CAD build for the part. Positions are in the model's coordinates, mm. A direction names the side the tool comes from. Round coordinates to 2 decimals unless told otherwise and drop trailing zeros. Loops run counter-clockwise (first coordinate to the right, second up) from the corner with the lowest first, then second, coordinate; pieces in that order, holes last.
Autodesk Fusion 360 part; units mm, degrees
sketch "Sketch1" plane through (0, 0, 0) normal (0, 0, 1) x (1, 0, 0)
  circle A0 centre (0, 0) radius 16
  circle A1 centre (0, 0) radius 12 construction
  line L0 (0, 0) -> (0, 16) construction
  circle A2 centre (0, 12) radius 2
  circle A3 centre (-12, 0) radius 2
  circle A4 centre (0, -12) radius 2
  circle A5 centre (12, 0) radius 2
  circle A6 centre (0, 0) radius 4
  dimension "d1" = 32
  dimension "d2" = 24
  dimension "d3" = 4
  dimension "d5" = 360
  dimension "d6" = 8
extrude "Extrude1" add sketch "Sketch1" along normal blind 3
sketch "Sketch2" plane through (0, 0, 3) normal (0, 0, 1) x (-1, 0, 0)
  circle A0 centre (0, -12) radius 2
  circle A1 centre (12, 0) radius 2
  circle A2 centre (0, 12) radius 2
  circle A3 centre (-12, 0) radius 2
  circle A4 centre (0, 0) radius 4
  circle A5 centre (0, 0) radius 16
  circle A6 centre (0, 0) radius 8
  dimension "d9" = 16
extrude "Extrude2" add sketch "Sketch2" along normal blind 10 contours A6
ref_plane "WorkPlane1" through (5.6569, -5.6569, 11.1327) normal (0.7071, -0.7071, 0) x (-0.7071, -0.7071, 0)
sketch "Sketch3" plane through (5.6569, -5.6569, 0) normal (0.7071, -0.7071, 0) x (-0.7071, -0.7071, 0)
  line L0 (-8, -13) -> (8, -13)
  line L1 (8, -3) -> (-8, -3)
  line L2 (0, -13) -> (0, -3) construction
  circle A0 centre (0, -8) radius 2
  line L3 (0, -8) -> (0, -10)
  dimension "d13" = 4
  dimension "d14" = 3
extrude "Extrude3" cut sketch "Sketch3" against normal blind 18
Item 1: Probe line 1 (Y direction, x = 0, z = 1.85); line 2 (X direction, y = 0, z = 7). List the from-to ranges inside material, lowest first.
Answers follow:
line 1: y = -16 to -14, -10 to -4, 4 to 10, 14 to 16
line 2: x = -8 to -4, 4 to 8
Item 2: Two-plate mould, pull along Y, no slides. Class faces 3 (the flat face through (4, 2, 13)), 4 (the cylindrical face through (-7.63, 2.4, 7.93)), 5 (the cylindrical face through (-4, 4, 10)): released by +Y, released by -Y, zero draft, split by the parting line, or undercut.
Answers follow:
face 3: zero draft
face 4: split by the parting line
face 5: undercut
Item 3: Cut at C-C, the plane z = 2.5. Give the cut face in (x, y).
Answers follow:
outline: circle Ø32 at (0, 0); hole circle Ø4 at (-12, 0); hole circle Ø8 at (0, 0); hole circle Ø4 at (0, -12); hole circle Ø4 at (0, 12); hole circle Ø4 at (12, 0)
Item 4: Flat gauge pins, fed straight in: P1, Ø6.5, axis at x = 0, y = -12, coming from the +Z side; P2, Ø3, axis at y = 6, z = 8, coming from the -X side; P3, Ø6, axis at x = 3.5, z = 5, coming from the -Y side. Where does each tip first touch, or does it go through?
Answers follow:
P1: stops at z = 3
P2: stops at x = -4.54
P3: stops at y = -15.95
Item 5: Cut at B-B, the plane x = 12. Give the cut face in (y, z).
Answers follow:
outline: (-10.58, 0) - (-2, 0) - (-2, 3) - (-10.58, 3) - close; (2, 0) - (10.58, 0) - (10.58, 3) - (2, 3) - close
Item 6: 3-axis set-ups, long thin cutter, end or side, ignore diameter. For faces 1 (the cylindrical face through (0, -14, 1)), 2 (the flat face through (-7.3, 3.8, 3)): which of +Z, -Z, +X, -X, +Y, -Y reach the whole face in a straight line?
Answers follow:
face 1: +Z, -Z
face 2: +Z
